Verification items for the finished model (mm, model axes). Face numbers are marked on the shaded views. Coordinates: 2 decimals unless noted, no trailing zeros. Order: outer loops, then holes, each group sorted by start corner. A loop starts at its lowest first (then second) coordinate and runs counter-clockwise, first axis right, second up.
Q1. Cross-section at A-A, the plane y = 44.5. Record the boundary of the cut face in (x, z), and give its area (3 significant figures).
Q2. Draft check along Z on the marked faces 1, 2, 3 and 4. Enter one of: pulls with the +Z half, pulls with the -Z half, needs draft (parallel to the pull), parting line crosses it, or undercut.
Q3. Cross-section at C-C, the plane z = 38. Record the boundary of the cut face in (x, y), and give its area (3 significant figures).
Q4. Cross-section at D-D, the plane y = 24. Record the boundary of the cut face in (x, z).
Q5. Cross-section at B-B, the plane z = -31. Record the boundary of the cut face in (x, y).
Q6. Thickness scan on line 1 (Z direction, x = -0.5, y = 41.5); line 2 (X direction, y = 19, z = -31); line 3 (X direction, y = 15.75, z = 0). Record the ranges inside material, lowest first.
Q7. Depth check by flat-ended pin: P1, Ø8, axis at x = 5.5, y = 39, coming from the -Z side; P2, Ø6.5, axis at x = 4, y = 4.5, coming from the -Z side; P3, Ø5, axis at x = 9.5, y = 27.5, coming from the -Z side; P4, Ø2, axis at x = -3, z = 61, coming from the -Y side. Enter the tip coordinate at first touch or a pass-through.
from build123d import *

# Parameters (mm, degrees)
BOSS_EXTRUDE1_DEPTH       = 18
CUT_EXTRUDE1_DEPTH        = 43
SKETCH3_W                 = 20
SKETCH3_H                 = 20
CUT_EXTRUDE4_DEPTH        = 8
SKETCH5_R                 = 4.5
CUT_EXTRUDE5_DEPTH        = 47
CUT_EXTRUDE6_DEPTH        = 55
F_6_0MM_DOWEL_HOLE1_D     = 6
F_6_0MM_DOWEL_HOLE1_DEPTH = 6
F_6_0MM_DOWEL_HOLE1_TIP   = 1.802581857
FILLET1_R                 = 6
FILLET2_R                 = 6


with BuildPart() as part:
    # Sketch1 → Boss-Extrude1 (new body, symmetric)
    with BuildSketch(Plane(origin=(0, 0, 0), x_dir=(0, 0, -1), z_dir=(1, 0, 0))):
        with BuildLine():
            Line((-82, 0), (82, 0))
            Line((82, 0), (79, 11))
            Line((79, 11), (50, 11))
            Line((50, 11), (50, 54))
            Line((50, 54), (22, 54))
            Line((22, 54), (22, 41))
            Line((22, 41), (19, 41))
            Line((19, 41), (19, 38))
            ThreePointArc((19, 38), (0, 19), (-19, 38))
            Line((-19, 38), (-19, 41))
            Line((-19, 41), (-22, 41))
            Line((-22, 41), (-22, 54))
            Line((-22, 54), (-50, 54))
            Line((-50, 54), (-50, 11))
            Line((-50, 11), (-79, 11))
            Line((-79, 11), (-82, 0))
        make_face()
    extrude(amount=BOSS_EXTRUDE1_DEPTH, both=True)

    # Sketch2 → Cut-Extrude1 (cut)
    with BuildSketch(Plane(origin=(0, 54, 0), x_dir=(1, 0, 0), z_dir=(0, 1, 0))):
        with BuildLine():
            Line((-18, 50), (-18, 44.497190923))
            ThreePointArc((-18, 44.497190923), (0, 48), (18, 44.497190923))
            Line((18, 44.497190923), (18, 50))
            Line((18, 50), (-18, 50))
        make_face()
        with BuildLine():
            Line((18, -50), (18, -44.497190923))
            ThreePointArc((18, -44.497190923), (0, -48), (-18, -44.497190923))
            Line((-18, -44.497190923), (-18, -50))
            Line((-18, -50), (18, -50))
        make_face()
    extrude(amount=-CUT_EXTRUDE1_DEPTH, mode=Mode.SUBTRACT)

    # Sketch3 → Cut-Extrude4 (cut)
    with BuildSketch(Plane(origin=(0, 0, 0), x_dir=(-1, 0, 0), z_dir=(0, -1, 0))):
        with Locations((0, 31)):
            Rectangle(SKETCH3_W, SKETCH3_H)
        with Locations((0, -31)):
            Rectangle(SKETCH3_W, SKETCH3_H)
    extrude(amount=-CUT_EXTRUDE4_DEPTH, mode=Mode.SUBTRACT)

    # Sketch5 → Cut-Extrude5 (cut, through all)
    with BuildSketch(Plane(origin=(0, 8, 0), x_dir=(-1, 0, 0), z_dir=(0, -1, 0))):
        with Locations(Location((0, 31, 0), (0, 0, 90))):  # turned: the seam where the file's is
            Circle(SKETCH5_R)
        with Locations(Location((0, -31, 0), (0, 0, 270))):  # turned: the seam where the file's is
            Circle(SKETCH5_R)
    extrude(amount=-CUT_EXTRUDE5_DEPTH, mode=Mode.SUBTRACT)

    # Sketch6 → Cut-Extrude6 (cut, through all)
    with BuildSketch(Plane(origin=(0, 0, 0), x_dir=(-1, 0, 0), z_dir=(0, -1, 0))):
        with BuildLine():
            Line((-4.5, 60.5), (-4.5, 67.5))
            ThreePointArc((-4.5, 67.5), (0, 72), (4.5, 67.5))
            Line((4.5, 67.5), (4.5, 60.5))
            ThreePointArc((4.5, 60.5), (0, 56), (-4.5, 60.5))
        make_face()
        with BuildLine():
            Line((-4.5, -60.5), (-4.5, -67.5))
            ThreePointArc((-4.5, -67.5), (0, -72), (4.5, -67.5))
            Line((4.5, -67.5), (4.5, -60.5))
            ThreePointArc((4.5, -60.5), (0, -56), (-4.5, -60.5))
        make_face()
    extrude(amount=-CUT_EXTRUDE6_DEPTH, mode=Mode.SUBTRACT)

    # Ø6.0mm Dowel Hole1
    with Locations(Plane.ZX.offset(19)):
        with Locations((0, 0)):
            Hole(F_6_0MM_DOWEL_HOLE1_D / 2, depth=F_6_0MM_DOWEL_HOLE1_DEPTH)
            with Locations((0, 0, -(F_6_0MM_DOWEL_HOLE1_DEPTH + F_6_0MM_DOWEL_HOLE1_TIP / 2))):  # 118° drill point
                Cone(0, F_6_0MM_DOWEL_HOLE1_D / 2, F_6_0MM_DOWEL_HOLE1_TIP, mode=Mode.SUBTRACT)

    # Fillet1
    fillet1_edges = [part.edges().sort_by_distance(p)[0] for p in [
        (0, 11, 48),
    ]]
    fillet(fillet1_edges, radius=FILLET1_R)

    # Fillet2
    fillet2_edges = [part.edges().sort_by_distance(p)[0] for p in [
        (0, 11, -48),
    ]]
    fillet(fillet2_edges, radius=FILLET2_R)


solid = part.part
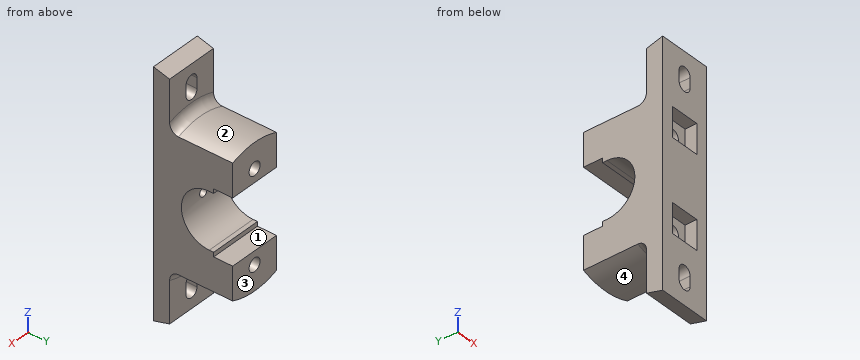
Check values:
1. outline: (-18, -44.5) arc R48 ccw to (18, -44.5) - (18, -22) - (-18, -22) - close; (-18, 22) - (18, 22) - (18, 44.5) arc R48 ccw to (-18, 44.5) - close; hole circle Ø9 at (0, -31); hole circle Ø9 at (0, 31)
1. area: 1,660 mm2
2. face 1: undercut
2. face 2: pulls with the +Z half
2. face 3: needs draft
2. face 4: pulls with the -Z half
3. outline: (-18, 0) - (-10, 0) - (-10, 8) - (10, 8) - (10, 0) - (18, 0) - (18, 54) - (-18, 54) - close
3. area: 1,780 mm2
4. outline: (-18, -44.5) arc R48 ccw to (18, -44.5) - (18, -12.85) - (-18, -12.85) - close; (-18, 12.85) - (18, 12.85) - (18, 44.5) arc R48 ccw to (-18, 44.5) - close; hole circle Ø9 at (0, -31); hole circle Ø9 at (0, 31)
5. outline: (-18, 0) - (-10, 0) - (-10, 8) - (-4.5, 8) - (-4.5, 54) - (-18, 54) - close; (4.5, 8) - (10, 8) - (10, 0) - (18, 0) - (18, 54) - (4.5, 54) - close
6. line 1: z = -48 to -35.47, -26.53 to -22, 22 to 26.53, 35.47 to 48
6. line 2: x = -18 to -4.5, 4.5 to 18
6. line 3: x = -18 to -3, 3 to 18
7. P1: stops at z = -47.98
7. P2: stops at z = -81.66
7. P3: stops at z = -47.49
7. P4: passes through
